Source: CAD feature listing. Evaluate the final solid. Frame: model axes, mm. A direction names the side the tool comes from. Coordinates: 2 decimals unless noted, no trailing zeros. Loops run counter-clockwise (first coordinate to the right, second up) from the corner with the lowest first, then second, coordinate; pieces in that order, holes last.
Item 1: Pull-direction query (X, two-part tool) for faces 1 (the cylindrical face through (0.468, 13.708, -1.878)), 2 (the cylindrical face through (-0.678, 12.807, 4.561)), 3 (the flat face through (10.1, 8.2, -3.81)); classes: +X half, -X half, draft (parallel to the pull), parting line (faces both ways), or undercut.
Item 2: Reachability of faces 4 (the cylindrical face through (0.462, 13.117, 6.261)), 5 (the flat face through (-0.619, -13, -2)) from +Z, -Z, +X, -X, +Y, -Y: full face, straight path, thin tool, end or side. Return the list, or none.
Item 3: Pin query (flat end, axial travel): pin 1 Ø1 at (x, z) = (-10.5, 6.5) entering from +Y; pin 2 Ø1.5 at (x, y) = (7.5, 8.5) entering from -Z; pin 3 Ø8 at (y, z) = (7.5, -1.5) entering from +X; pin 4 Ø8 at (x, z) = (4.5, 5.5) entering from -Y. Return the tip coordinate at first contact, or that it passes through.
Item 4: Section query A-A, the plane y = 0. Return the cut outline in (x, z) (3 decimals).
Item 5: Line query: probe 1 along X at (y, z) = (0, 0.75) (3 decimals); probe 2 along Y at (x, z) = (6.25, 4.25); probe 3 along Y at (x, z) = (6, -2.5). Output: solid intervals per line, ascending.
Item 6: Section query B-B, the plane x = 7. Return the cut outline in (y, z), then the cut area to 3 significant figures.
Item 7: Section query C-C, the plane z = 7.5. Return the cut outline in (x, y) (3 decimals), then the cut area to 3 significant figures.
```python
from build123d import *

# Parameters (mm, degrees)
F1_DEPTH = 12.7
F2_DEPTH = 3.81


with BuildPart() as f1:
    # F0 (on Top) → F1 (new body)
    with BuildSketch(Plane.XY):
        with BuildLine():
            ThreePointArc((-0.619034, -12.810052), (-0.124602, 12.824395), (0.867818, -12.795605))
            Line((0.867818, -12.795605), (0.867818, -13.096279))
            ThreePointArc((0.867818, -13.096279), (-0.104246, 13.124586), (-0.659679, -13.108411))
            Line((-0.659679, -13.108411), (-0.619034, -12.810052))
        make_face()
    extrude(amount=F1_DEPTH)

    # F0 (on Top) → F2 (join)
    with BuildSketch(Plane.XY):
        with BuildLine():
            Line((0.867818, -13.096279), (0.867818, -12.795605))
            Line((0.867818, -12.795605), (0.826493, -13.098952))
            ThreePointArc((0.826493, -13.098952), (0.847157, -13.097631), (0.867818, -13.096279))
        make_face()
        with BuildLine():
            ThreePointArc((-0.619034, -12.810052), (-0.124602, 12.824395), (0.867818, -12.795605))
            Line((0.867818, -12.795605), (0.867818, -13.096279))
            ThreePointArc((0.867818, -13.096279), (-0.104246, 13.124586), (-0.659679, -13.108411))
            Line((-0.659679, -13.108411), (-0.619034, -12.810052))
        make_face()
        with BuildLine():
            Line((-0.619034, -13.702024), (-0.619034, -12.810052))
            Line((-0.619034, -12.810052), (-0.659679, -13.108411))
            ThreePointArc((-0.659679, -13.108411), (-0.104246, 13.124586), (0.867818, -13.096279))
            Line((0.867818, -13.096279), (0.867818, -13.688519))
            ThreePointArc((0.867818, -13.688519), (-0.124575, 13.715434), (-0.619034, -13.702024))
        make_face()
    extrude(amount=-F2_DEPTH)


solid = f1.part
```
Verdict:
1. face 1: parting line
1. face 2: undercut
1. face 3: draft
2. face 4: +Z
2. face 5: +Z, -Z, -Y
3. pin 1: stops at y = 8.5
3. pin 2: passes through
3. pin 3: stops at x = 13.26
3. pin 4: stops at y = -13.1
4. outline: (-13.716, -3.81) - (-12.825, -3.81) - (-12.825, 12.7) - (-13.125, 12.7) - (-13.125, 0) - (-13.716, 0) - close; (12.825, -3.81) - (13.716, -3.81) - (13.716, 0) - (13.125, 0) - (13.125, 12.7) - (12.825, 12.7) - close
5. probe 1: x = -13.125 to -12.825, 12.825 to 13.125
5. probe 2: y = -11.54 to -11.2, 11.2 to 11.54
5. probe 3: y = -12.33 to -11.33, 11.33 to 12.33
6. outline: (-11.8, -3.81) - (-10.75, -3.81) - (-10.75, 12.7) - (-11.1, 12.7) - (-11.1, 0) - (-11.8, 0) - close; (10.75, -3.81) - (11.8, -3.81) - (11.8, 0) - (11.1, 0) - (11.1, 12.7) - (10.75, 12.7) - close
6. area: 17.0 mm2
7. outline: (-0.66, -13.108) - (-0.619, -12.81) arc R12.825 cw (long way) to (0.868, -12.796) - (0.868, -13.096) arc R13.125 ccw (long way) to start
7. area: 24.0 mm2
